Can you work these out from the model? Positions are in its coordinate system, mm. A direction names the side the tool comes from. Give positions to 0.01 mm unless a question says otherwise; leave off trailing zeros. Write each loop counter-clockwise with the first axis right and the second up, starting at its lowest first coordinate (ties: lowest second). Pieces come first, ordered by that corner, then holes. Notation, with made-up numbers: M 20.25,-0.75 L 79.25,-0.75 A25 cw 79.25,32.25 Z; hole C 17,29 d9. An arc over 180 degrees is marked long. Write each question's results on one line, items separated by ' | '.
Autodesk Inventor part; units mm, degrees
ref_plane "YZ Plane" through (0, 0, 0) normal (1, 0, 0) x (0, 1, 0)
ref_plane "XZ Plane" through (0, 0, 0) normal (0, 1, 0) x (-1, 0, 0)
ref_plane "XY Plane" through (0, 0, 0) normal (0, 0, 1) x (1, 0, 0)
sketch "Sketch1" plane through (0, 0, 0) normal (0, 1, 0) x (-1, 0, 0)
  circle A0 centre (0, -35) radius 25
  line L0 (0, 0) -> (50, 0)
  line L1 (50, 0) -> (-50, 0)
  line L2 (21.4679, -47.8113) -> (50, 0)
  line L3 (-21.4679, -47.8113) -> (-50, 0)
  circle A1 centre (0, -35) radius 3
  dimension "d4" = 50
  dimension "d5" = 50
  dimension "d6" = 100
  dimension "d7" = 6
extrude "Extrusion1" add sketch "Sketch1" along normal blind 10
sketch "Sketch2" plane through (-50, 0, 0) normal (0, 0, 1) x (1, 0, 0)
  line L0 (0, 10) -> (100, 10)
  line L1 (0, 10) -> (50, 10)
  line L2 (50, 10) -> (50, 0)
  circle A0 centre (35, 5) radius 1
  circle A1 centre (65, 5) radius 1
  dimension "d11" = 2
  dimension "d12" = 2
extrude "Extrusion2" cut sketch "Sketch2" against normal blind 10
properties part number "stojan2"
Item 1: Thinking about a two-plate mould opening in Z: for faces 3 (the face through (0, 5, -38)), 4 (the face through (15, 5, -10)), 5 (the face through (-35.534, 4.93, -24.24)), which applies, +Z half, -Z half, draft (parallel to the pull), parting line (faces both ways), or undercut?
Geometry says:
face 3: undercut | face 4: +Z half | face 5: -Z half
Item 2: I'm going to push flat-ended pins straight in: pin 1 (1.5 mm diameter, centred on y = 5, z = -31, fed in from -X); pin 2 (4 mm diameter, centred on y = 3, z = -38, fed in from +X); pin 3 (1.8 mm diameter, centred on x = 15, y = 5, fed in from -Z); pin 4 (7 mm diameter, centred on x = 0, z = -35, fed in from +Y). Where does each tip first touch, or does it pass through?
Geometry says:
pin 1: stops at x = -31.95 | pin 2: stops at x = 28.52 | pin 3: stops at z = -55.64 | pin 4: stops at y = 10
Item 3: If I drill on line 1 (Y direction, x = 15, z = -2); line 2 (Z direction, x = 0, y = 7.75); line 3 (Z direction, x = -1, y = 5), over which ranges is the centre line in solid material (lowest first)? Write a range as from..to.
Geometry says:
line 1: y = 0..4, 6..10 | line 2: z = -60..-38, -32..0 | line 3: z = -59.98..-37.83, -32.17..0
Item 4: I want a section at C-C, the plane x = -15. Please give me the cut outline in (y, z), and give its area (3 significant figures).
Geometry says:
outline: M 0,-55 L 10,-55 L 10,0 L 6,0 L 6,-10 L 4,-10 L 4,0 L 0,0 Z | area: 530 mm2
Item 5: I want a section at D-D, the plane z = -14. Please give me the cut outline in (x, y), and give its area (3 significant figures).
Geometry says:
outline: M -41.65,0 L 41.65,0 L 41.65,10 L -41.65,10 Z | area: 833 mm2
Item 6: For faces 1 (the face through (35.534, 4.93, -24.24)), 2 (the face through (-14, 5, -5)), which set-ups out of +Z, -Z, +X, -X, +Y, -Y let a thin tool reach every point of the face, with its end or its side?
Geometry says:
face 1: -Z, +X, +Y, -Y | face 2: +Z
Item 7: I want a section at B-B, the plane y = 9. Please give me the cut outline in (x, z).
Geometry says:
outline: M -50,0 L -21.47,-47.81 A25 ccw 21.47,-47.81 L 50,0 Z; hole C 0,-35 d6
Item 8: I want a section at A-A, the plane x = 0. Please give me the cut outline in (y, z).
Geometry says:
outline: M 0,-60 L 10,-60 L 10,-38 L 0,-38 Z; M 0,-32 L 10,-32 L 10,0 L 0,0 Z
